```python
from build123d import *

# Parameters (mm, degrees)
SKETCH_1_R          = 1.625
EXTRUDE_1_DEPTH     = 3
FILLET_1_R          = 10
SKETCH_3_R          = 1.625
CUT_EXTRUDE_1_DEPTH = 10
CUT_EXTRUDE_4_DEPTH = 10


with BuildPart() as part:
    # Эскиз1 → Бобышка-Вытянуть1 (new body)
    with BuildSketch(Plane.XY):
        with BuildLine():
            ThreePointArc((-32.5, 4), (-35.328427125, -2.828427125), (-28.5, 0))
            Line((-28.5, 0), (28.5, 0))
            ThreePointArc((28.5, 0), (35.328427125, -2.828427125), (32.5, 4))
            Line((32.5, 4), (32.5, 24.5))
            ThreePointArc((32.5, 24.5), (35.328427125, 31.328427125), (28.5, 28.5))
            Line((28.5, 28.5), (-28.5, 28.5))
            ThreePointArc((-28.5, 28.5), (-35.328427125, 31.328427125), (-32.5, 24.5))
            Line((-32.5, 24.5), (-32.5, 4))
        make_face()
        with Locations((-32.5, 0)):
            Circle(SKETCH_1_R, mode=Mode.SUBTRACT)
        with Locations((32.5, 28.5)):
            Circle(SKETCH_1_R, mode=Mode.SUBTRACT)
        with Locations((-32.5, 28.5)):
            Circle(SKETCH_1_R, mode=Mode.SUBTRACT)
        with Locations((32.5, 0)):
            Circle(SKETCH_1_R, mode=Mode.SUBTRACT)
    extrude(amount=EXTRUDE_1_DEPTH)

    # Скругление1
    fillet_1_edges = [part.edges().sort_by_distance(p)[0] for p in [
        (28.5, 0, 1.5),
        (-28.5, 0, 1.5),
        (-32.5, 4, 1.5),
        (-32.5, 24.5, 1.5),
        (-28.5, 28.5, 1.5),
        (28.5, 28.5, 1.5),
        (32.5, 24.5, 1.5),
        (32.5, 4, 1.5),
    ]]
    fillet(fillet_1_edges, radius=FILLET_1_R)

    # Эскиз3 → Вырез-Вытянуть1 (cut)
    with BuildSketch(Plane(origin=(0, 0, 0), x_dir=(-1, 0, 0), z_dir=(0, 0, -1))):
        with Locations((-17.5, 25)):
            Circle(SKETCH_3_R)
        with Locations(Location((17.5, 25, 0), (0, 0, 180))):
            Circle(SKETCH_3_R)
    extrude(amount=-CUT_EXTRUDE_1_DEPTH, mode=Mode.SUBTRACT)

    # Эскиз7 → Вырез-Вытянуть4 (cut)
    with BuildSketch(Plane.XY.offset(3)):
        with BuildLine():
            Line((-20, 20.5), (20, 20.5))
            ThreePointArc((20, 20.5), (26, 14.5), (20, 8.5))
            Line((20, 8.5), (-20, 8.5))
            ThreePointArc((-20, 8.5), (-26, 14.5), (-20, 20.5))
        make_face()
    extrude(amount=-CUT_EXTRUDE_4_DEPTH, mode=Mode.SUBTRACT)


solid = part.part
```
Check sheet for the modelled part. Datum: model origin and axes. Units: mm. A direction names the side the tool comes from. Give positions to 0.01 mm unless a question says otherwise; leave off trailing zeros. Write each loop counter-clockwise with the first axis right and the second up, starting at its lowest first coordinate (ties: lowest second). Pieces come first, ordered by that corner, then holes. Notation, with made-up numbers: (73, 44) - (86, 44) arc R26 ccw to (86, 68) - close; hole circle Ø2 at (-26.75, 43.25). An arc over 180 degrees is marked (long way). Answer as a JSON object with one key per item and string values. Group by question number.
1) Sectioned sample at A-A (z = 1.4). Record the cut outline in (x, y) (3 decimals).
2) Release check for a two-part mould opening along Y. For faces 4 (the face through (-1, 6, 3)), 5 (the face through (35.39, 31.266, 1.479)), 6 (the face through (-26.53, -0.76, 1.52)) record: pulls with the +Y half, pulls with the -Y half, needs draft (parallel to the pull), parting line crosses it, or undercut.
3) Thickness scan on probe 1 along Y at (x, z) = (17.5, 1.55) (3 decimals); probe 2 along Y at (x, z) = (-6, 2); probe 3 along Y at (x, z) = (-32, 0.3). Record the ranges inside material, lowest first. Write a range as from..to.
4) Sectioned sample at B-B (x = 17.5). Record the cut outline in (y, z) (3 decimals), then the cut area to 4 significant figures.
5) Sectioned sample at C-C (y = 14.5). Record the cut outline in (x, z), then the cut area to 3 significant figures.
6) Depth check by flat-ended pin: P1, Ø2.5, axis at x = 17.5, y = 25, coming from the -Z side; P2, Ø5, axis at x = 32.5, y = 0, coming from the -Z side; P3, Ø1, axis at x = -2, z = 1.5, coming from the -Y side; P4, Ø0.9, axis at y = 13.5, z = 1, coming from the +X side. Enter the tip coordinate at first touch or a pass-through.
7) Access from +Z, -Z, +X, -X, +Y, -Y to the whole of each face (thin tool, end or side, straight path). Record for faces 1 (the face through (0, 28.5, 1)), 2 (the face through (-33.22, 22.43, 1.52)), 3 (the face through (33.26, 5.97, 1.52)).
8) Sectioned sample at D-D (y = 25). Record the cut outline in (x, z) (3 decimals), then the cut area to 3 significant figures.
Geometry results:
{
 "1": {"outline": "(-35.357, 2.799) arc R4 ccw to (-29.701, -2.857) arc R10 cw to (-22.702, 0) - (22.702, 0) arc R10 cw to (29.701, -2.857) arc R4 ccw to (35.357, 2.799) arc R10 cw to (32.5, 9.798) - (32.5, 18.702) arc R10 cw to (35.357, 25.701) arc R4 ccw to (29.701, 31.357) arc R10 cw to (22.702, 28.5) - (-22.702, 28.5) arc R10 cw to (-29.701, 31.357) arc R4 ccw to (-35.357, 25.701) arc R10 cw to (-32.5, 18.702) - (-32.5, 9.798) arc R10 cw to start; hole circle Ø3.25 at (-32.5, 0); hole circle Ø3.25 at (-32.5, 28.5); hole (-20, 8.5) - (20, 8.5) arc R6 ccw to (20, 20.5) - (-20, 20.5) arc R6 ccw to start; hole circle Ø3.25 at (-17.5, 25); hole circle Ø3.25 at (17.5, 25); hole circle Ø3.25 at (32.5, 0); hole circle Ø3.25 at (32.5, 28.5)"},
 "2": {"face 4": "needs draft", "face 5": "undercut", "face 6": "pulls with the -Y half"},
 "3": {"probe 1": "y = 0..8.5, 20.5..23.375, 26.625..28.5", "probe 2": "y = 0..8.5, 20.5..28.5", "probe 3": "y = -3.97..-1.55, 1.55..26.95, 30.05..32.47"},
 "4": {"outline": "(0, 0) - (8.5, 0) - (8.5, 3) - (0, 3) - close; (20.5, 0) - (23.375, 0) - (23.375, 3) - (20.5, 3) - close; (26.625, 0) - (28.5, 0) - (28.5, 3) - (26.625, 3) - close", "area": "39.75 mm^2"},
 "5": {"outline": "(-32.5, 0) - (-26, 0) - (-26, 3) - (-32.5, 3) - close; (26, 0) - (32.5, 0) - (32.5, 3) - (26, 3) - close", "area": "39.0 mm^2"},
 "6": {"P1": "passes through", "P2": "stops at z = 0", "P3": "stops at y = 0", "P4": "stops at x = 32.5"},
 "7": {"face 1": "+Z, -Z, +Y", "face 2": "+Z, -Z, -X", "face 3": "+Z, -Z, +X"},
 "8": {"outline": "(-34.732, 0) - (-19.125, 0) - (-19.125, 3) - (-34.732, 3) - close; (-15.875, 0) - (15.875, 0) - (15.875, 3) - (-15.875, 3) - close; (19.125, 0) - (34.732, 0) - (34.732, 3) - (19.125, 3) - close", "area": "189 mm^2"}
}
